```python
from build123d import *

# Parameters (mm, degrees)
BOSS_EXTRUDE4_DEPTH   = 12.7
F_8_CLEARANCE_HOLE1_D = 4.9149
FILLET2_R             = 4.7625
FILLET3_R             = 12.7
M6_CLEARANCE_HOLE2_D  = 7
BOSS_EXTRUDE5_START   = -19.558
BOSS_EXTRUDE5_DEPTH   = 25.908
CUT_EXTRUDE1_START    = -6.35
CUT_EXTRUDE1_DEPTH    = 6.35
CUT_EXTRUDE2_START    = -25.908
CUT_EXTRUDE2_DEPTH    = 6.35


with BuildPart() as part:
    # Sketch7 → Boss-Extrude4 (new, symmetric)
    with BuildSketch(Plane.XY):
        Polygon((-12.954, -19.05), (-12.954, 12.954), (-6.604, 12.954), (-6.604, 38.1), (6.604, 38.1), (6.604, 12.954), (12.954, 12.954), (12.954, -19.05), (9.779, -19.05), (9.779, 9.779), (-9.779, 9.779), (-9.779, -19.05), align=None)
    extrude(amount=BOSS_EXTRUDE4_DEPTH, both=True)

    # #8 Clearance Hole1 (through all)
    with Locations(Plane(origin=(12.954, 0, 0), x_dir=(0, 0, -1), z_dir=(1, 0, 0))):
        with Locations((-6.985, -14.2875), (6.985, -14.2875)):
            Hole(F_8_CLEARANCE_HOLE1_D / 2)

    # Fillet2
    fillet2_edges = [part.edges().sort_by_distance(p)[0] for p in [
        (11.3665, -19.05, -12.7),
        (-11.3665, -19.05, -12.7),
        (-11.3665, -19.05, 12.7),
        (11.3665, -19.05, 12.7),
    ]]
    fillet(fillet2_edges, radius=FILLET2_R)

    # Fillet3
    fillet3_edges = [part.edges().sort_by_distance(p)[0] for p in [
        (0, 38.1, 12.7),
        (0, 38.1, -12.7),
    ]]
    fillet(fillet3_edges, radius=FILLET3_R - 0.0001)  # a hair under: the kernel refuses the full size

    # M6 Clearance Hole2 (through all)
    with Locations(Plane(origin=(-6.604, 0, 0), x_dir=(0, 0, -1), z_dir=(-1, 0, 0))):
        with Locations((0, -25.4)):
            Hole(M6_CLEARANCE_HOLE2_D / 2)

    # Sketch12 → Boss-Extrude5 (add)
    with BuildSketch(Plane(origin=(6.604, 0, 0), x_dir=(0, 0, -1), z_dir=(1, 0, 0)).offset(BOSS_EXTRUDE5_START)):
        with BuildLine():
            Line((-12.7, 12.954), (-12.7, 21.807897552))
            ThreePointArc((-12.7, 21.807897552), (-12.481567114, 22.059395027), (-12.201960784, 21.878330933))
            ThreePointArc((-12.201960784, 21.878330933), (-8.610950381, 16.065037036), (-2.52726809, 12.954))
            Line((-2.52726809, 12.954), (-12.7, 12.954))
        make_face()
        with BuildLine():
            Line((12.7, 12.954), (12.7, 21.807897552))
            ThreePointArc((12.7, 21.807897552), (12.481567114, 22.059395027), (12.201960784, 21.878330933))
            ThreePointArc((12.201960784, 21.878330933), (8.610950381, 16.065037036), (2.52726809, 12.954))
            Line((2.52726809, 12.954), (12.7, 12.954))
        make_face()
    extrude(amount=BOSS_EXTRUDE5_DEPTH)

    # Sketch13 → Cut-Extrude1 (cut)
    with BuildSketch(Plane(origin=(12.954, 0, 0), x_dir=(0, 0, -1), z_dir=(1, 0, 0)).offset(CUT_EXTRUDE1_START)):
        with BuildLine():
            Line((-2.52726809, 12.954), (2.52726809, 12.954))
            ThreePointArc((2.52726809, 12.954), (0, 12.7), (-2.52726809, 12.954))
        make_face()
    extrude(amount=CUT_EXTRUDE1_DEPTH, mode=Mode.SUBTRACT)

    # Sketch13<2> → Cut-Extrude2 (cut)
    with BuildSketch(Plane(origin=(12.954, 0, 0), x_dir=(0, 0, -1), z_dir=(1, 0, 0)).offset(CUT_EXTRUDE2_START)):
        with BuildLine():
            Line((-2.52726809, 12.954), (2.52726809, 12.954))
            ThreePointArc((2.52726809, 12.954), (0, 12.7), (-2.52726809, 12.954))
        make_face()
    extrude(amount=CUT_EXTRUDE2_DEPTH, mode=Mode.SUBTRACT)


solid = part.part
```
Could you check a few things on this model? Use its own coordinates, in mm. A direction names the side the tool comes from. Round coordinates to 2 decimals unless told otherwise and drop trailing zeros. Write each loop counter-clockwise with the first axis right and the second up, starting at its lowest first coordinate (ties: lowest second). Pieces come first, ordered by that corner, then holes. Notation, with made-up numbers: M -18,26 L -3,26 A17 cw -3,33 Z; hole C 59.25,-2 d9. An arc over 180 degrees is marked long. Answer in a Markdown table with one row per item. Add a question column.
Q1. Imagine slicing it at A-A (y = -6). Please give me the cut outline in (x, z).
Q2. Imagine slicing it at D-D (y = 19.5). Please give me the cut outline in (x, z).
Q3. If we mould it in two halves opening along X, with no side actions, what happens to faces 3 (the flat face through (0, 10, -12.7)), 4 (the flat face through (6.604, 23, -3)), 5 (the flat face through (9.779, -5, 0)), 6 (the flat face through (-9.779, -4, 0))? For each: +X half, -X half, draft (parallel to the pull), parting line (faces both ways), or undercut.
Q4. Will these pins go through, and if not, where does the flat tip stop? pin 1 Ø4 at (y, z) = (-14.29, 6.98) entering from -X; pin 2 Ø2 at (x, z) = (-5.5, 1) entering from -Y; pin 3 Ø6 at (x, z) = (0, 9.5) entering from +Y; pin 4 Ø2 at (y, z) = (21.5, -7.5) entering from -X.
Q5. If I drill on line 1 (X direction, y = 6.5, z = -9.75); line 2 (Z direction, x = 1, y = 25.4); line 3 (X direction, y = 27, z = 11.25), over which ranges is the centre line in solid material (lowest first)? Write a range as from..to.
Q6. Imagine slicing it at C-C (x = -10.5). Give the number of separate pieces and of enclosed holes in the cut face, then the cut area to 3 significant figures.
Q7. On a 3-axis mill with a long thin cutter (end or side, diameter ignored), from which of +Z, -Z, +X, -X, +Y, -Y can I reach the whole of each face in a straight line? I mean faces 1 (the cylindrical face through (11.344, -16.468, 8.119)), 2 (the flat face through (0, 9.779, 0)). Say none if no direction works.
Values:
| question | item | result |
|---|---|---|
| 1 | outline | M -12.95,-12.7 L -9.78,-12.7 L -9.78,12.7 L -12.95,12.7 Z; M 9.78,-12.7 L 12.95,-12.7 L 12.95,12.7 L 9.78,12.7 Z |
| 2 | outline | M -12.95,-12.7 L 12.95,-12.7 L 12.95,-11.25 L 6.6,-11.25 L 6.6,11.25 L 12.95,11.25 L 12.95,12.7 L -12.95,12.7 L -12.95,11.25 L -6.6,11.25 L -6.6,-11.25 L -12.95,-11.25 Z |
| 3 | face 3 | draft |
| 3 | face 4 | +X half |
| 3 | face 5 | undercut |
| 3 | face 6 | undercut |
| 4 | pin 1 | through |
| 4 | pin 2 | y = 9.78 |
| 4 | pin 3 | y = 36.31 |
| 4 | pin 4 | x = -6.6 |
| 5 | line 1 | -12.95..-9.78, 9.78..12.95 |
| 5 | line 2 | -12.7..-3.5, 3.5..12.7 |
| 5 | line 3 | -6.6..6.6 |
| 6 | separate pieces | 1 |
| 6 | enclosed holes | 2 |
| 6 | area | 827 mm^2 |
| 7 | face 1 | +X, -X |
| 7 | face 2 | +Z, -Z, -Y |
